from build123d import *

# Parameters (mm, degrees)
SKETCH1_W                       = 160
SKETCH1_H                       = 75
BOSS_EXTRUDE1_DEPTH             = 4
F_3_0MM_DOWEL_HOLE1_D           = 3
F_3_0MM_DOWEL_HOLE2_D           = 3
F_3_0MM_PRESS_DOWEL_HOLE1_D     = 3
F_3_0MM_PRESS_DOWEL_HOLE1_DEPTH = 6
F_3_0MM_PRESS_DOWEL_HOLE1_TIP   = 0.901290929


with BuildPart() as part:
    # Sketch1 → Boss-Extrude1 (new body)
    with BuildSketch(Plane.XY):
        with Locations((80, 37.5)):
            Rectangle(SKETCH1_W, SKETCH1_H)
    extrude(amount=BOSS_EXTRUDE1_DEPTH)

    # Ø3.0mm Dowel Hole1 (through all)
    with Locations(Plane.XY.offset(4)):
        with Locations((16.5, 52.5), (16.5, 22.5), (143.5, 52.5), (143.5, 22.5)):
            Hole(F_3_0MM_DOWEL_HOLE1_D / 2)

    # Ø3.0mm Dowel Hole2 (through all)
    with Locations(Plane.XY.offset(4)):
        with Locations((16.5, 37.5), (143.5, 37.5)):
            Hole(F_3_0MM_DOWEL_HOLE2_D / 2)

    # Ø3.0mm Press Dowel Hole1
    with Locations(Plane.XY.offset(4)):
        with Locations((44.446877451, 15), (44.446877451, 55)):
            Hole(F_3_0MM_PRESS_DOWEL_HOLE1_D / 2, depth=F_3_0MM_PRESS_DOWEL_HOLE1_DEPTH)
            with Locations((0, 0, -(F_3_0MM_PRESS_DOWEL_HOLE1_DEPTH + F_3_0MM_PRESS_DOWEL_HOLE1_TIP / 2))):  # 118° drill point
                Cone(0, F_3_0MM_PRESS_DOWEL_HOLE1_D / 2, F_3_0MM_PRESS_DOWEL_HOLE1_TIP, mode=Mode.SUBTRACT)


solid = part.part
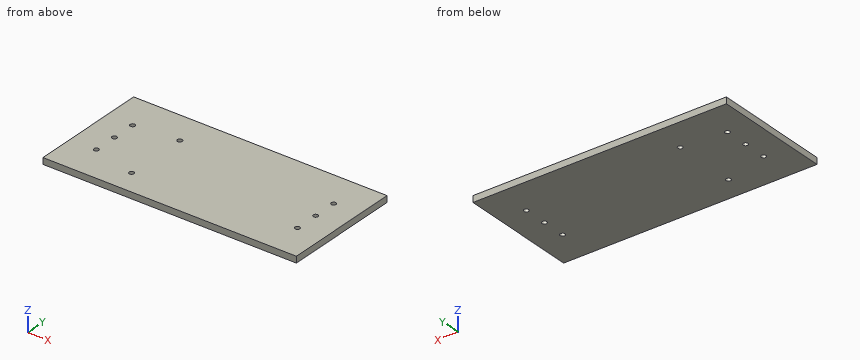
CAD build for the part. Positions are in the model's coordinates, mm. Give positions to 0.01 mm unless a question says otherwise; leave off trailing zeros. Order: outer loops, then holes, each group sorted by start corner. A loop starts at its lowest first (then second) coordinate and runs counter-clockwise, first axis right, second up. Notation, with made-up numbers: (84.25, 35.5) - (95.25, 35.5) arc R28 ccw to (95.25, 67.5) - close; hole circle Ø1 at (-29, 34). An arc over 180 degrees is marked (long way). Answer in a Markdown table with one row per item.
1. Saw through at B-B, the plane y = 15. Give the cut face in (x, z), plus the area to 3 significant figures.
Data:
| item | result |
|---|---|
| outline | (0, 0) - (42.95, 0) - (42.95, 4) - (0, 4) - close; (45.95, 0) - (160, 0) - (160, 4) - (45.95, 4) - close |
| area | 628 mm² |
2. Saw through at C-C, the plane y = 37.5. Give the cut face in (x, z).
Data:
| item | result |
|---|---|
| outline | (0, 0) - (15, 0) - (15, 4) - (0, 4) - close; (18, 0) - (142, 0) - (142, 4) - (18, 4) - close; (145, 0) - (160, 0) - (160, 4) - (145, 4) - close |
3. Saw through at A-A, the plane x = 143.5. Give the cut face in (y, z).
Data:
| item | result |
|---|---|
| outline | (0, 0) - (21, 0) - (21, 4) - (0, 4) - close; (24, 0) - (36, 0) - (36, 4) - (24, 4) - close; (39, 0) - (51, 0) - (51, 4) - (39, 4) - close; (54, 0) - (75, 0) - (75, 4) - (54, 4) - close |
4. Probe probe 1 along Y at (x, z) = (143.5, 3.2); probe 2 along Y at (x, z) = (144.5, 1.6). List the from-to ranges inside material, lowest first. Write a range as [from, to].
Data:
| item | result |
|---|---|
| probe 1 | y = [0, 21], [24, 36], [39, 51], [54, 75] |
| probe 2 | y = [0, 21.38], [23.62, 36.38], [38.62, 51.38], [53.62, 75] |
5. Flat gauge pin, fed straight in: pin 1 (2.5 mm diameter, centred on x = 44.45, y = 15, fed in from -Z). Where does the tip first touch, or does it go through?
Data:
| item | result |
|---|---|
| pin 1 | passes through |
